Read the model definition and answer for the solid it produces. Units are mm, in the model's axes. A direction names the side the tool comes from. Give positions to 0.01 mm unless a question says otherwise; leave off trailing zeros. Order: outer loops, then holes, each group sorted by start corner. A loop starts at its lowest first (then second) coordinate and runs counter-clockwise, first axis right, second up. Notation, with made-up numbers: (71.25, 0) - (95.25, 0) arc R27 cw to (95.25, 37) - close; hole circle Ø9 at (-22, -37.5). An arc over 180 degrees is marked (long way). Write each question's results on one line, items separated by ' | '.
from build123d import *

# Parameters (mm, degrees)
SKETCH_1_R          = 15
EXTRUDE_1_DEPTH     = 3
SKETCH_2_R          = 7.95
EXTRUDE_2_DEPTH     = 3.5
SKETCH_3_R          = 0.9
EXTRUDE_3_DEPTH     = 2
SKETCH_4_R          = 2
SKETCH_4_R_2        = 0.9
CUT_EXTRUDE_1_DEPTH = 3
CHAMFER_1_SIZE      = 0.5


with BuildPart() as part:
    # 草图1 → 凸台-拉伸1 (new body)
    with BuildSketch(Plane(origin=(0, 0, 0), x_dir=(1, 0, 0), z_dir=(0, 1, 0))):
        Circle(SKETCH_1_R)
    extrude(amount=EXTRUDE_1_DEPTH)

    # 草图2 → 凸台-拉伸2 (add)
    with BuildSketch(Plane(origin=(0, 3, 0), x_dir=(1, 0, 0), z_dir=(0, 1, 0))):
        Circle(SKETCH_2_R)
    extrude(amount=EXTRUDE_2_DEPTH)

    # 草图3 → 凸台-拉伸3 (add)
    with BuildSketch(Plane(origin=(0, 6.5, 0), x_dir=(1, 0, 0), z_dir=(0, 1, 0))):
        Circle(SKETCH_3_R)
    extrude(amount=EXTRUDE_3_DEPTH)

    # 草图4 → 切除-拉伸1 (cut)
    with BuildSketch(Plane(origin=(0, 6.5, 0), x_dir=(1, 0, 0), z_dir=(0, 1, 0))):
        Circle(SKETCH_4_R)
        Circle(SKETCH_4_R_2, mode=Mode.SUBTRACT)
    extrude(amount=-CUT_EXTRUDE_1_DEPTH, mode=Mode.SUBTRACT)

    # 倒角1
    chamfer_1_edges = [part.edges().sort_by_distance(p)[0] for p in [
        (-2, 6.5, 0),
    ]]
    chamfer(chamfer_1_edges, length=CHAMFER_1_SIZE)


solid = part.part
(1) Section B-B (z = 0) is taken. Give the vertices of the cut face in (x, y).
Conclusion:
outline: (-15, 0) - (15, 0) - (15, 3) - (7.95, 3) - (7.95, 6.5) - (2.5, 6.5) - (2, 6) - (2, 3.5) - (0.9, 3.5) - (0.9, 8.5) - (-0.9, 8.5) - (-0.9, 3.5) - (-2, 3.5) - (-2, 6) - (-2.5, 6.5) - (-7.95, 6.5) - (-7.95, 3) - (-15, 3) - close
(2) Section D-D (y = 2) is taken. Give the vertices of the cut face in (x, z).
Conclusion:
outline: circle Ø30 at (0, 0)
(3) The mould has two halves that part along X. Classify faces 3 (the face through (-1.72, 4.73, 7.76)), 4 (the face through (0, 0, 0)), 5 (the face through (0, 5, 2)): pulls with the +X half, pulls with the -X half, needs draft (parallel to the pull), parting line crosses it, or undercut.
Conclusion:
face 3: parting line crosses it | face 4: needs draft | face 5: undercut
(4) For faces 1 (the face through (-14.985, 1.479, -0.66)), 2 (the face through (0.86, 6.04, -0.27)), determine the directions among +Z, -Z, +X, -X, +Y, -Y from which every point of the face is accessible in a straight line to the end or side of a thin tool.
Conclusion:
face 1: +Y, -Y | face 2: +Y
(5) Section C-C (x = 0) is taken. Give the vertices of the cut face in (y, z), plus the area to 3 significant figures.
Conclusion:
outline: (0, -15) - (3, -15) - (3, -7.95) - (6.5, -7.95) - (6.5, -2.5) - (6, -2) - (3.5, -2) - (3.5, -0.9) - (8.5, -0.9) - (8.5, 0.9) - (3.5, 0.9) - (3.5, 2) - (6, 2) - (6.5, 2.5) - (6.5, 7.95) - (3, 7.95) - (3, 15) - (0, 15) - close | area: 142 mm^2
(6) Section A-A (y = 4.75) is taken. Give the vertices of the cut face in (x, z).
Conclusion:
outline: circle Ø15.9 at (0, 0); circle Ø1.8 at (0, 0); hole circle Ø4 at (0, 0)
(7) Consider probe 1 along Z at (x, y) = (0, 5.05); probe 2 along Y at (x, z) = (12, 5.5). Determine where each line is inside the solid, lowest interval first. Write a range as [from, to].
Conclusion:
probe 1: [-7.95, -2], [-0.9, 0.9], [2, 7.95] | probe 2: [0, 3]
(8) Each of these flat-tipped pins is pushed along its axis until it touches: pin 1 (1 mm diameter, centred on y = 6.5, z = -1, fed in from +X); pin 2 (2 mm diameter, centred on x = 3, z = 9, fed in from +Y); pin 3 (1 mm diameter, centred on y = 2, z = 9, fed in from +X). Where does it stop, or does it pass through?
Conclusion:
pin 1: x = 7.93 | pin 2: y = 3 | pin 3: x = 12.36
